from build123d import *

# Parameters (mm, degrees)
F0_W     = 210
F0_H     = 297
F0_W_2   = 28
F0_H_2   = 63
F1_DEPTH = 25


with BuildPart() as f1:
    # F0 (on Front) → F1 (new body)
    with BuildSketch(Plane.XZ):
        Rectangle(F0_W, F0_H)
        with Locations((-59.5, -90)):
            Rectangle(F0_W_2, F0_H_2, mode=Mode.SUBTRACT)
        with Locations((0, -108)):
            Rectangle(F0_W_2, F0_H_2, mode=Mode.SUBTRACT)
        with Locations((59.5, -90)):
            Rectangle(F0_W_2, F0_H_2, mode=Mode.SUBTRACT)
        with Locations((0, -36)):
            Rectangle(F0_W_2, F0_H_2, mode=Mode.SUBTRACT)
        with Locations((-59.5, 0)):
            Rectangle(F0_W_2, F0_H_2, mode=Mode.SUBTRACT)
        with Locations((-59.5, 90)):
            Rectangle(F0_W_2, F0_H_2, mode=Mode.SUBTRACT)
        with Locations((0, 36)):
            Rectangle(F0_W_2, F0_H_2, mode=Mode.SUBTRACT)
        with Locations((59.5, 0)):
            Rectangle(F0_W_2, F0_H_2, mode=Mode.SUBTRACT)
        with Locations((0, 108)):
            Rectangle(F0_W_2, F0_H_2, mode=Mode.SUBTRACT)
        with Locations((59.5, 90)):
            Rectangle(F0_W_2, F0_H_2, mode=Mode.SUBTRACT)
    extrude(amount=F1_DEPTH)


solid = f1.part
Read the model definition and answer for the solid it produces. Units are mm, in the model's axes. Coordinates: 2 decimals unless noted, no trailing zeros. Order: outer loops, then holes, each group sorted by start corner. A loop starts at its lowest first (then second) coordinate and runs counter-clockwise, first axis right, second up. Notation, with made-up numbers: M -24,28.5 L -17,28.5 A29 ccw -17,53.5 Z; hole C -19,40.25 d2. An arc over 180 degrees is marked long. Put each result on its own line as item: value. Start each with the question number.
Item 1: Section D-D, the plane y = -17.75 is taken. Count the separate pieces of the cut face and the enclosed holes in it, plus the area to 3 significant figures.
Item 2: The mould has two halves that part along X. Classify faces 1 (the face through (0, -12, 76.5)), 2 (the face through (105, -12, -2)), 3 (the face through (-1, 0, 2)): +X half, -X half, draft (parallel to the pull), parting line (faces both ways), or undercut.
Item 3: Consider probe 1 along Z at (x, y) = (72, -18.5); probe 2 along X at (y, z) = (-23.25, 69.5); probe 3 along Z at (x, y) = (-9, -19). Determine where each line is inside the solid, lowest interval first. Write a range as [from, to].
Item 4: Section A-A, the plane z = 46.5 is taken. Determine the outline of the cut face in (x, y).
Item 5: Section C-C, the plane x = -8 is taken. Determine the outline of the cut face in (y, z), plus the area to 4 significant figures.
Item 6: Section B-B, the plane x = 58 is taken. Determine the outline of the cut face in (y, z).
Computed:
1. separate pieces: 1
1. enclosed holes: 10
1. area: 44,700 mm2
2. face 1: undercut
2. face 2: +X half
2. face 3: draft
3. probe 1: z = [-148.5, -121.5], [-58.5, -31.5], [31.5, 58.5], [121.5, 148.5]
3. probe 2: x = [-105, -73.5], [-45.5, 45.5], [73.5, 105]
3. probe 3: z = [-148.5, -139.5], [-76.5, -67.5], [-4.5, 4.5], [67.5, 76.5], [139.5, 148.5]
4. outline: M -105,-25 L -14,-25 L -14,0 L -105,0 Z; M 14,-25 L 105,-25 L 105,0 L 14,0 Z
5. outline: M -25,-148.5 L 0,-148.5 L 0,-139.5 L -25,-139.5 Z; M -25,-76.5 L 0,-76.5 L 0,-67.5 L -25,-67.5 Z; M -25,-4.5 L 0,-4.5 L 0,4.5 L -25,4.5 Z; M -25,67.5 L 0,67.5 L 0,76.5 L -25,76.5 Z; M -25,139.5 L 0,139.5 L 0,148.5 L -25,148.5 Z
5. area: 1,125 mm2
6. outline: M -25,-148.5 L 0,-148.5 L 0,-121.5 L -25,-121.5 Z; M -25,-58.5 L 0,-58.5 L 0,-31.5 L -25,-31.5 Z; M -25,31.5 L 0,31.5 L 0,58.5 L -25,58.5 Z; M -25,121.5 L 0,121.5 L 0,148.5 L -25,148.5 Z
